```python
from build123d import *

# Parameters (mm, degrees)
SKETCH1_R           = 85
SKETCH1_R_2         = 1.5
BOSS_EXTRUDE1_DEPTH = 10
BOSS_EXTRUDE2_DEPTH = 5


with BuildPart() as part:
    # Sketch1 → Boss-Extrude1 (new body)
    with BuildSketch(Plane.XY):
        Circle(SKETCH1_R)
        with Locations((0, 80)):
            Circle(SKETCH1_R_2, mode=Mode.SUBTRACT)
        with Locations((69.282032303, 40)):
            Circle(SKETCH1_R_2, mode=Mode.SUBTRACT)
        with Locations((69.282032303, -40)):
            Circle(SKETCH1_R_2, mode=Mode.SUBTRACT)
        with Locations((0, -80)):
            Circle(SKETCH1_R_2, mode=Mode.SUBTRACT)
        with Locations((-69.282032303, -40)):
            Circle(SKETCH1_R_2, mode=Mode.SUBTRACT)
        with Locations((-69.282032303, 40)):
            Circle(SKETCH1_R_2, mode=Mode.SUBTRACT)
    extrude(amount=BOSS_EXTRUDE1_DEPTH)

    # Sketch2 → Boss-Extrude2 (add, symmetric)
    with BuildSketch(Plane(origin=(0, 0, 0), x_dir=(1, 0, 0), z_dir=(0, 1, 0))):
        Polygon((-50, 0), (-45, 0), (-45, 2), (45, 2), (45, 0), (50, 0), (50, 4), (-50, 4), align=None)
    extrude(amount=BOSS_EXTRUDE2_DEPTH, both=True)


solid = part.part
```
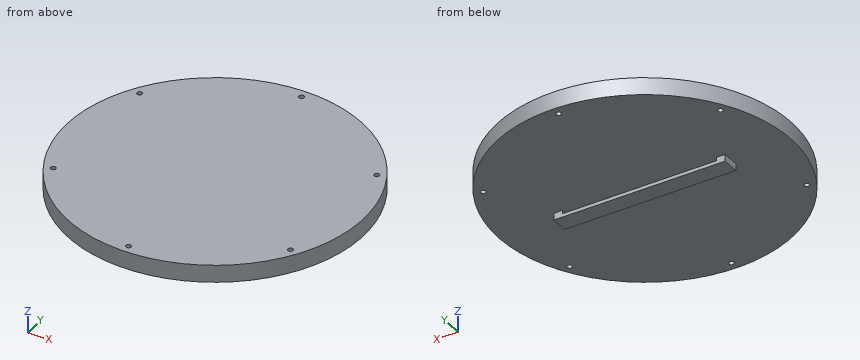
The listing builds one solid part. Answer for the finished solid, in the listing's coordinates (mm). Give positions to 0.01 mm unless a question says otherwise; leave off trailing zeros. Write each loop counter-clockwise with the first axis right and the second up, starting at its lowest first coordinate (ties: lowest second). Pieces come first, ordered by that corner, then holes. Notation, with made-up numbers: (-15.75, 6.5) -> (-11.75, 6.5) arc R18 cw to (-11.75, 14.5) -> close; hole circle Ø9 at (-10.5, 68.5). An arc over 180 degrees is marked (long way). Use one line per item in the form item = value.
1) Section C-C on x = -36.5 is taken. Write down the section's boundary in (y, z).
Result:
outline = (-76.76, 0) -> (76.76, 0) -> (76.76, 10) -> (-76.76, 10) -> close; (-5, -4) -> (5, -4) -> (5, -2) -> (-5, -2) -> close
2) Section D-D on y = 48.5 is taken. Write down the section's boundary in (x, z), plus the area to 3 significant figures.
Result:
outline = (-69.81, 0) -> (69.81, 0) -> (69.81, 10) -> (-69.81, 10) -> close
area = 1,400 mm²
3) Section B-B on z = 5.75 is taken. Write down the section's boundary in (x, y), plus the area to 3 significant figures.
Result:
outline = circle Ø170 at (0, 0); hole circle Ø3 at (-69.28, -40); hole circle Ø3 at (-69.28, 40); hole circle Ø3 at (0, -80); hole circle Ø3 at (0, 80); hole circle Ø3 at (69.28, -40); hole circle Ø3 at (69.28, 40)
area = 22,700 mm²
4) Straight lines are drawn through the part: probe 1 along Y at (x, z) = (0, 5.75); probe 2 along Z at (x, y) = (-18.5, 36); probe 3 along X at (y, z) = (-51.5, 8). For each, find the intervals that lie inside material, in ascending order.
Result:
probe_1 = -85 to -81.5, -78.5 to 78.5, 81.5 to 85
probe_2 = 0 to 10
probe_3 = -67.62 to 67.62
5) Section A-A on y = 0 is taken. Write down the section's boundary in (x, z).
Result:
outline = (-85, 0) -> (-50, 0) -> (-50, -4) -> (50, -4) -> (50, 0) -> (85, 0) -> (85, 10) -> (-85, 10) -> close; hole (-45, -2) -> (45, -2) -> (45, 0) -> (-45, 0) -> close
6) Each of these flat-tipped pins is pushed along its axis until it touches: P1, Ø5, axis at x = -27, z = -0.5, coming from the +Y side; P2, Ø1.6, axis at y = 1, z = -0.5, coming from the +X side; P3, Ø5, axis at x = -69.28, y = -40, coming from the +Z side; P4, Ø3, axis at y = 17, z = -0.5, coming from the -X side. Where does it stop, or does it pass through?
Result:
P1 = 81.38
P2 = 85
P3 = 10
P4 = -83.56
